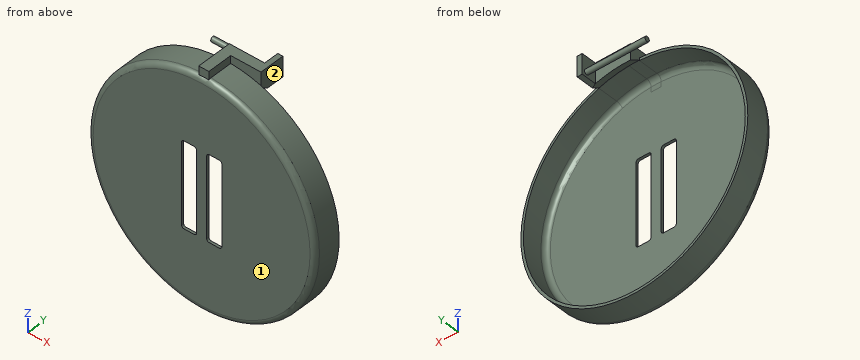
```python
from build123d import *

# Parameters (mm, degrees)
SKETCH1_R                = 22.5
SKETCH1_R_2              = 22
BOSS_EXTRUDE1_DEPTH      = 5
SKETCH3_R                = 22.5
BOSS_EXTRUDE2_DEPTH      = 0.5
SKETCH6_W                = 3
SKETCH6_H                = 17
CUT_EXTRUDE1_DEPTH       = 10
CUT_EXTRUDE1_DEPTH_BACK  = 10
FILLET1_R                = 0.5
FILLET3_R                = 1
SKETCH7_W                = 2
SKETCH7_H                = 4
BOSS_EXTRUDE3_DEPTH      = 2
BOSS_EXTRUDE3_DEPTH_BACK = 5
SKETCH8_W                = 4
SKETCH8_H                = 2
BOSS_EXTRUDE4_DEPTH      = 6
SKETCH9_W                = 1
SKETCH9_H                = 4
BOSS_EXTRUDE5_DEPTH      = 3
SKETCH10_R               = 0.5
BOSS_EXTRUDE6_DEPTH      = 12


with BuildPart() as part:
    # Sketch1 → Boss-Extrude1 (new body)
    with BuildSketch(Plane(origin=(0, 0, 0), x_dir=(1, 0, 0), z_dir=(0, 1, 0))):
        with Locations(Location((0, 0, 0), (0, 0, 270))):
            Circle(SKETCH1_R)
        with Locations(Location((0, 0, 0), (0, 0, 270))):
            Circle(SKETCH1_R_2, mode=Mode.SUBTRACT)
    extrude(amount=BOSS_EXTRUDE1_DEPTH)

    # Sketch3 → Boss-Extrude2 (add)
    with BuildSketch(Plane(origin=(0, 0, 0), x_dir=(1, 0, 0), z_dir=(0, 1, 0))):
        with Locations(Location((0, 0, 0), (0, 0, 270))):
            Circle(SKETCH3_R)
    extrude(amount=-BOSS_EXTRUDE2_DEPTH)

    # Sketch6 → Cut-Extrude1 (cut, two sides)
    with BuildSketch(Plane.XZ.offset(0.5)) as cut_extrude1_sk:
        with Locations((2.5, 0)):
            Rectangle(SKETCH6_W, SKETCH6_H)
        with Locations((-2.5, 0)):
            Rectangle(SKETCH6_W, SKETCH6_H)
    extrude(amount=CUT_EXTRUDE1_DEPTH, mode=Mode.SUBTRACT)
    extrude(cut_extrude1_sk.sketch, amount=-CUT_EXTRUDE1_DEPTH_BACK, mode=Mode.SUBTRACT)

    # Fillet1
    fillet1_edges = [part.edges().sort_by_distance(p)[0] for p in [
        (-4, -0.25, 8.5),
        (-4, -0.25, -8.5),
        (-1, -0.25, -8.5),
        (-1, -0.25, 8.5),
        (1, -0.25, 8.5),
        (1, -0.25, -8.5),
        (4, -0.25, -8.5),
        (4, -0.25, 8.5),
    ]]
    fillet(fillet1_edges, radius=FILLET1_R)

    # Fillet3
    fillet3_edges = [part.edges().sort_by_distance(p)[0] for p in [
        (0, 0, -22),
        (0, -0.5, -22.5),
    ]]
    fillet(fillet3_edges, radius=FILLET3_R)

    # Sketch7 → Boss-Extrude3 (add, two sides)
    with BuildSketch(Plane(origin=(0, 5, 0), x_dir=(1, 0, 0), z_dir=(0, 1, 0))) as boss_extrude3_sk:
        with Locations((0, -22)):
            Rectangle(SKETCH7_W, SKETCH7_H)
    extrude(amount=BOSS_EXTRUDE3_DEPTH)
    extrude(boss_extrude3_sk.sketch, amount=-BOSS_EXTRUDE3_DEPTH_BACK)

    # Sketch8 → Boss-Extrude4 (add)
    with BuildSketch(Plane(origin=(1, 0, 0), x_dir=(0, 0, -1), z_dir=(1, 0, 0))):
        with Locations((-22, 6)):
            Rectangle(SKETCH8_W, SKETCH8_H)
    extrude(amount=BOSS_EXTRUDE4_DEPTH)

    # Sketch9 → Boss-Extrude5 (add)
    with BuildSketch(Plane(origin=(0, 7, 0), x_dir=(1, 0, 0), z_dir=(0, 1, 0))):
        with Locations((6.5, -22)):
            Rectangle(SKETCH9_W, SKETCH9_H)
    extrude(amount=BOSS_EXTRUDE5_DEPTH)

    # Sketch10 → Boss-Extrude6 (add)
    with BuildSketch(Plane.ZY.offset(-6)):
        with Locations(Location((21, 9, 0), (0, 0, 180))):
            Circle(SKETCH10_R)
    extrude(amount=BOSS_EXTRUDE6_DEPTH)

    # Sketch12 → Cut-Revolve1 (revolve, cut)
    with BuildSketch(Plane(origin=(0, 0, 0), x_dir=(0, 0, -1), z_dir=(1, 0, 0)), mode=Mode.PRIVATE) as cut_revolve1_sk:
        with BuildLine():
            Line((-18, 12), (-22, 5.07179677))
            Line((-22, 5.07179677), (-22, 1))
            ThreePointArc((-22, 1), (-21.707106781, 0.292893219), (-21, 0))
            Line((-21, 0), (0, 0))
            Line((0, 0), (0, 12))
            Line((0, 12), (-18, 12))
        make_face()
    revolve(cut_revolve1_sk.sketch.rotate(Axis((0, 12.625, 0), (0, -1, 0)), 341.446995465), axis=Axis((0, 12.625, 0), (0, -1, 0)), mode=Mode.SUBTRACT)


solid = part.part
```
Work out the finished part from the listing and answer in its coordinate system (mm). Face numbers are marked on the shaded views. A direction names the side the tool comes from. Give positions to 0.01 mm unless a question says otherwise; leave off trailing zeros. Order: outer loops, then holes, each group sorted by start corner. A loop starts at its lowest first (then second) coordinate and runs counter-clockwise, first axis right, second up.
1. For the marked faces 1 and 2, determine the directions among +Z, -Z, +X, -X, +Y, -Y from which every point of the face is accessible in a straight line to the end or side of a thin tool.
Result sheet:
face 1: +Z, -Z, +X, -X, -Y
face 2: +Z, -Z, +X, +Y
2. Section A-A, the plane z = 0 is taken. Determine the outline of the cut face in (x, y).
Result sheet:
outline: (-22.5, 0.5) arc R1 ccw to (-21.5, -0.5) - (-4, -0.5) - (-4, 0) - (-21, 0) arc R1 cw to (-22, 1) - (-22, 5) - (-22.5, 5) - close; (-1, -0.5) - (1, -0.5) - (1, 0) - (-1, 0) - close; (4, -0.5) - (21.5, -0.5) arc R1 ccw to (22.5, 0.5) - (22.5, 5) - (22, 5) - (22, 1) arc R1 cw to (21, 0) - (4, 0) - close
3. Section C-C, the plane y = 1.75 is taken. Determine the outline of the cut face in (x, z), and give its area (3 significant figures).
Result sheet:
outline: (-1, 22.48) arc R22.5 ccw (long way) to (1, 22.48) - (1, 24) - (-1, 24) - close; hole circle Ø44 at (0, 0)
area: 72.9 mm2
4. Section B-B, the plane x = 0 is taken. Determine the outline of the cut face in (y, z), and give its area (3 significant figures).
Result sheet:
outline: (-0.5, -21.5) arc R1 ccw to (0.5, -22.5) - (5, -22.5) - (5, -22) - (1, -22) arc R1 cw to (0, -21) - (0, 21) arc R1 cw to (1, 22) - (5.07, 22) - (7, 20.89) - (7, 24) - (0, 24) - (0, 22.37) arc R1 ccw to (-0.5, 21.5) - close; circle Ø1 at (9, 21)
area: 40.9 mm2
5. Each of these flat-tipped pins is pushed along its axis until it touches: P1, Ø6, axis at x = -2.5, z = -5, coming from the +Y side; P2, Ø1.3, axis at x = 3.5, z = 23.5, coming from the -Y side; P3, Ø6, axis at y = 4, z = 5.5, coming from the -X side. Where does it stop, or does it pass through?
Result sheet:
P1: stops at y = 0
P2: stops at y = 5
P3: stops at x = -22.36
6. Straight lines are drawn through the part: L1, parallel to Z at x = 0, y = 3.5; L2, parallel to X at y = 2.65, z = 0; L3, parallel to Y at x = 7, z = -10. For each, find the intervals that lie inside material, in ascending order.
Result sheet:
L1: z = -22.5 to -22, 22 to 24
L2: x = -22.5 to -22, 22 to 22.5
L3: y = -0.5 to 0
